```python
from build123d import *

# Parameters (mm, degrees)
EXTRUDE_1_DEPTH = 30
CHAMFER_1_SIZE  = 5
FILLET_1_R      = 10


with BuildPart() as part:
    # 草图1 → 凸台-拉伸1 (new, symmetric)
    with BuildSketch(Plane.XY):
        with BuildLine():
            Line((0, 0), (0, 55))
            Line((0, 55), (-30, 60))
            Line((-30, 60), (-30, 85))
            Line((-30, 85), (-0.286548804, 88.961793493))
            ThreePointArc((-0.286548804, 88.961793493), (31.348985254, 79.40804216), (45, 49.312677466))
            Line((45, 49.312677466), (45, 0))
            Line((45, 0), (0, 0))
        make_face()
    extrude(amount=EXTRUDE_1_DEPTH, both=True)

    # 倒角1
    chamfer_1_edges = [part.edges().sort_by_distance(p)[0] for p in [
        (0, 0, 0),
        (45, 0, 0),
        (22.5, 0, 30),
        (22.5, 0, -30),
    ]]
    chamfer(chamfer_1_edges, length=CHAMFER_1_SIZE)

    # 圆角1
    fillet_1_edges = [part.edges().sort_by_distance(p)[0] for p in [
        (-30, 60, 0),
    ]]
    fillet(fillet_1_edges, radius=FILLET_1_R)


solid = part.part
```
Geometry: final body of the model. Coordinates: model frame, mm. A direction names the side the tool comes from. Give positions to 0.01 mm unless a question says otherwise; leave off trailing zeros. Order: outer loops, then holes, each group sorted by start corner. A loop starts at its lowest first (then second) coordinate and runs counter-clockwise, first axis right, second up. Notation, with made-up numbers: (77, 6) -> (130, 6) arc R16 cw to (130, 27) -> close; hole circle Ø8 at (70, -39). An arc over 180 degrees is marked (long way). Write each question's results on one line, items separated by ' | '. Start each with the question number.
1) Section C-C (x = 28). Return loops of the section in (y, z).
2) Section B-B (y = 26.5). Return loops of the section in (x, z), then the cut area to 3 significant figures.
3) Section A-A (z = -2). Return loops of the section in (x, y).
4) Set-up query: faces 1 (the flat face through (0, 30, 0)), 2 (the flat face through (16, 48, 30)). Return all of +Z, -Z, +X, -X, +Y, -Y with unobstructed straight access to the full face (end or side cutting, diameter ignored); none if empty.
5) Line query: line 1 (X direction, y = 15, z = 16); line 2 (Y direction, x = -17, z = -17.5); line 3 (X direction, y = 64, z = 0). Output: solid intervals per line, ascending. Write a range as from..to.
6) First-contact query: pin 1 (15 mm diameter, centred on y = 27.5, z = -9, fed in from -X); pin 2 (4 mm diameter, centred on y = 67, z = -19.5, fed in from -X); pin 3 (12 mm diameter, centred on x = -18.5, z = 23, fed in from -Y); pin 4 (10 mm diameter, centred on x = 25, z = 11, fed in from +Y). Flat tips, straight axial feed; report the tip coordinate or a pass-through.
7) Section D-D (y = 62). Return loops of the section in (x, z).
Calculated:
1) outline: (0, -25) -> (5, -30) -> (82.04, -30) -> (82.04, 30) -> (5, 30) -> (0, 25) -> close
2) outline: (0, -30) -> (45, -30) -> (45, 30) -> (0, 30) -> close | area: 2,700 mm2
3) outline: (-30, 68.47) arc R10 ccw to (-21.64, 58.61) -> (0, 55) -> (0, 5) -> (5, 0) -> (40, 0) -> (45, 5) -> (45, 49.31) arc R40 ccw to (-0.29, 88.96) -> (-30, 85) -> close
4) face 1: +Z, -Z, -X, -Y | face 2: +Z, +X, -X, +Y, -Y
5) line 1: 0..45 | line 2: 57.83..86.73 | line 3: -28.94..42.21
6) pin 1: x = 0 | pin 2: x = -30 | pin 3: y = 57.08 | pin 4: y = 86.39
7) outline: (-27.62, -30) -> (42.93, -30) -> (42.93, 30) -> (-27.62, 30) -> close
